Autodesk Fusion 360 part; units mm, degrees
sketch "Sketch2" plane through (0, 0, 0) normal (0, 0, 1) x (1, 0, 0)
  line L0 (0, -19) -> (0, -17)
  line L1 (0, -17) -> (0, 22) construction
  line L2 (-22, 0) -> (25, 0) construction
  line L3 (0, 0) -> (5, 0)
  line L4 (20, 0) -> (20, 20)
  line L5 (0, 0) -> (20, 0)
  line L6 (20, 20) -> (17.5, 20)
  line L7 (17.5, 20) -> (17.5, 4.5)
  line L8 (17.5, 4.5) -> (9, 4.5)
  line L9 (9, 4.5) -> (9, 2)
  line L10 (9, 2) -> (0, 2)
  line L11 (0, 2) -> (0, 0)
  dimension "d76" = 20
  dimension "d77" = 20
  dimension "d78" = 2
  dimension "d79" = 4.5
  dimension "d80" = 17.5
  dimension "d81" = 9
revolve "Revolve1" add sketch "Sketch2" angle 360 about axis through (0, -17, 0) along (0, 1, 0)
sketch "Sketch3" plane through (0, 0, 0) normal (0, -1, 0) x (1, 0, 0)
  circle A0 centre (0, 0) radius 20
  line L0 (3, -19.7737) -> (3, 19.7737)
  circle A1 centre (0, 0) radius 20
  line L1 (0, 1.75) -> (0, 22.5)
  line L2 (-3, -19.7737) -> (-3, 19.7737)
  line L3 (-19.8431, 2.5) -> (-23, 2.5)
  arc A2 (-23, 2.5) -> (-23, -2.5) centre (-23, 0) ccw
  line L4 (-23, -2.5) -> (-19.8431, -2.5)
  line L5 (-15, 0) -> (-23, 0) construction
  arc A3 (23, -2.5) -> (23, 2.5) centre (23, 0) ccw
  line L6 (23, -2.5) -> (19.8431, -2.5)
  line L7 (15, 0) -> (23, 0) construction
  line L8 (19.8431, 2.5) -> (23, 2.5)
  circle A4 centre (-23, 0) radius 1.375
  circle A5 centre (23, 0) radius 1.375
  dimension "d83" = 6
  dimension "d84" = 5
  dimension "d88" = 2.75
extrude "Extrude4" cut sketch "Sketch3" against normal blind 17 from surface at -3 contours A0 L0 A1 L2
extrude "Extrude5" add sketch "Sketch3" against normal blind 3 contours A0 A1 A3 L6 L8 | A0 A1 L3 A2 L4
sketch "Sketch4" plane through (0, 0, 0) normal (0, 0, 1) x (1, 0, 0)
Here's how the part is built. I have some questions about the finished solid (model axes, mm). A direction names the side the tool comes from. Give positions to 0.01 mm unless a question says otherwise; leave off trailing zeros. Order: outer loops, then holes, each group sorted by start corner. A loop starts at its lowest first (then second) coordinate and runs counter-clockwise, first axis right, second up. Notation, with made-up numbers: M -31.5,38.25 L 1.5,38.25 A21 cw 1.5,57.25 Z; hole C -18,51.5 d2. An arc over 180 degrees is marked long. Answer as a JSON object with one key per item and string values. Group by question number.
1) Suppose I cut it at D-D, the plane z = -11.5. Write out the boundary of the cut face in (x, y), plus the area to 3 significant figures.
2) We'd pull the mould along Z, two halves only. Please class faces 1 (the flat face through (0, 3, -14)), 2 (the cylindrical face through (-24.374, 1.479, 0.06)), 3 (the flat face through (-21, 1, 2.5)): pulls with the +Z half, pulls with the -Z half, needs draft (parallel to the pull), parting line crosses it, or undercut.
3) I'm going to push flat-ended pins straight in: pin 1 Ø1.5 at (y, z) = (18, -6.5) entering from -X; pin 2 Ø1 at (y, z) = (13, -7) entering from -X; pin 3 Ø3.5 at (y, z) = (13, 13) entering from +X; pin 4 Ø2 at (x, z) = (-23, 0) entering from +Y. Where does each tip first touch, or does it pass through?
4) Please list where these lines run through material, in increasing order: L1, parallel to Z at x = 23, y = 0.7 (3 decimals); L2, parallel to X at y = 3.3, z = 0; L3, parallel to X at y = 3.25, z = 3. Write a range as [from, to].
5) Suppose I cut it at A-A, the plane y = 14.75. Write out the boundary of the cut face in (x, z).
6) On a 3-axis mill with a long thin cutter (end or side, diameter ignored), from which of +Z, -Z, +X, -X, +Y, -Y can I reach the whole of each face in a straight line? I mean faces 4 (the flat face through (-3, 10, -18)), 5 (the cylindrical face through (17.497, 12.142, -0.343)), 6 (the flat face through (21, 1, -2.5)). Say none if no direction works.
7) Suppose I cut it at C-C, the plane x = 0. Write out the boundary of the cut face in (y, z).
8) Suppose I cut it at B-B, the plane z = 0. Write out the boundary of the cut face in (x, y) (3 decimals), plus the area to 3 significant figures.
Results found:
{
 "1": {"outline": "M -16.36,0 L 16.36,0 L 16.36,20 L 13.19,20 L 13.19,4.5 L 3,4.5 L 3,3 L -3,3 L -3,4.5 L -13.19,4.5 L -13.19,20 L -16.36,20 Z", "area": "237 mm²"},
 "2": {"face 1": "needs draft", "face 2": "undercut", "face 3": "pulls with the +Z half"},
 "3": {"pin 1": "x = -19.16", "pin 2": "x = -18.91", "pin 3": "x = 16.54", "pin 4": "through"},
 "4": {"L1": "[-2.5, -1.375], [1.375, 2.5]", "L2": "[-20, -9], [9, 20]", "L3": "[-19.77, -8.49], [8.49, 19.77]"},
 "5": {"outline": "M -3,-19.77 L -3,-17.24 A17.5 cw -3,17.24 L -3,19.77 A20 ccw Z; M 3,-19.77 A20 ccw 3,19.77 L 3,17.24 A17.5 cw 3,-17.24 Z"},
 "6": {"face 4": "+Z, -Z, +Y", "face 5": "+Y", "face 6": "-Z, +X, +Y, -Y"},
 "7": {"outline": "M 0,-20 L 3,-20 L 3,-9 L 2,-9 L 2,9 L 3,9 L 3,20 L 0,20 Z"},
 "8": {"outline": "M -25.5,0 L -24.375,0 L -24.375,3 L -25.5,3 Z; M -21.625,0 L 21.625,0 L 21.625,3 L 20,3 L 20,20 L 17.5,20 L 17.5,4.5 L 9,4.5 L 9,2 L -9,2 L -9,4.5 L -17.5,4.5 L -17.5,20 L -20,20 L -20,3 L -21.625,3 Z; M 24.375,0 L 25.5,0 L 25.5,3 L 24.375,3 Z", "area": "229 mm²"}
}
